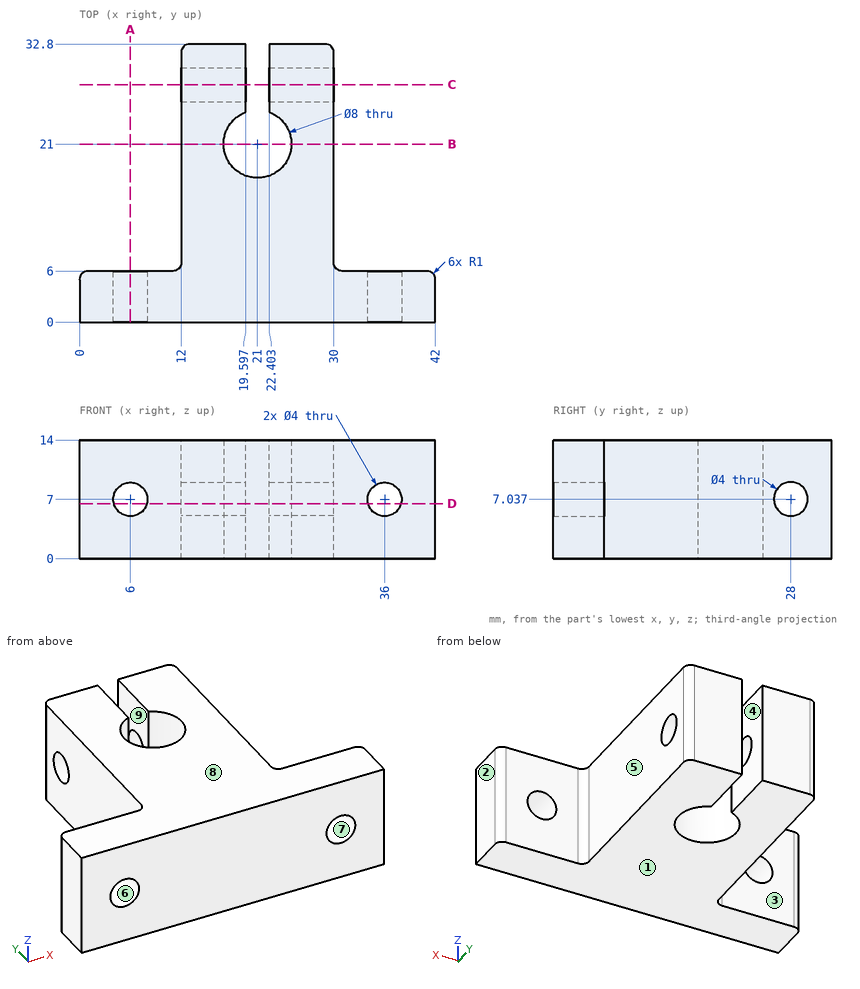
Print and shaded views of the part. All mm, measured from the part's lowest x, y and z. A direction names the side the tool comes from. Give positions to 0.01 mm unless a question says otherwise; leave off trailing zeros. Loops run counter-clockwise (first coordinate to the right, second up) from the corner with the lowest first, then second, coordinate; pieces in that order, holes last. Notation, with made-up numbers: M 4.25,-5 L 10.25,-5 A32 cw 10.25,28 Z; hole C 51,61 d1. An arc over 180 degrees is marked long. Write each question's results on one line, items separated by ' | '.
Q1. Band-saw the part on A-A on x = 6. Write the cut outline in (y, z), and give its area (3 significant figures).
Geometry check:
outline: M 0,0 L 6,0 L 6,5 L 0,5 Z; M 0,9 L 6,9 L 6,14 L 0,14 Z | area: 60.0 mm²
Q2. Mould opens along Z. For the marked faces 6, 7, 8 and 9 say: pulls with the +Z half, pulls with the -Z half, needs draft (parallel to the pull), parting line crosses it, or undercut.
Geometry check:
face 6: undercut | face 7: undercut | face 8: pulls with the +Z half | face 9: needs draft
Q3. Which spindle directions (+Z, -Z, +X, -X, +Y, -Y) get a long thin tool onto all of the face, cutting with end or side? Do the marked faces 1, 2, 3, 4 and 5. Say none if no direction does.
Geometry check:
face 1: -Z, +X, -X, +Y, -Y | face 2: +Z, -Z, +X, +Y, -Y | face 3: +Z, -Z, -X, +Y | face 4: +Z, -Z, +Y | face 5: +Z, -Z, +X, +Y
Q4. Flat gauge pins, fed straight in: P1, Ø8, axis at y = 18, z = 9, coming from the -X side; P2, Ø5, axis at x = 33.5, z = 8.5, coming from the +Y side; P3, Ø4.5, axis at y = 28, z = 7.04, coming from the +X side. Where does each tip first touch, or does it go through?
Geometry check:
P1: stops at x = 12 | P2: stops at y = 6 | P3: stops at x = 30
Q5. Band-saw the part on C-C on y = 28. Write the cut outline in (x, z), and give its area (3 significant figures).
Geometry check:
outline: M 12,0 L 19.6,0 L 19.6,5.04 L 12,5.04 Z; M 12,9.04 L 19.6,9.04 L 19.6,14 L 12,14 Z; M 22.4,0 L 30,0 L 30,5.04 L 22.4,5.04 Z; M 22.4,9.04 L 30,9.04 L 30,14 L 22.4,14 Z | area: 152 mm²
Q6. Band-saw the part on B-B on y = 21. Write the cut outline in (x, z).
Geometry check:
outline: M 12,0 L 17,0 L 17,14 L 12,14 Z; M 25,0 L 30,0 L 30,14 L 25,14 Z
Q7. Band-saw the part on D-D on z = 6.5. Give the number of separate pieces and of enclosed holes in the cut face.
Geometry check:
separate pieces: 5 | enclosed holes: 0
Q8. Probe probe 1 along X at (y, z) = (21, 10.5); probe 2 along Z at (x, y) = (6, 3.75); probe 3 along Y at (x, z) = (19, 7) (1 decimal). List the from-to ranges inside material, lowest first.
Geometry check:
probe 1: x = 12 to 17, 25 to 30 | probe 2: z = 0 to 5, 9 to 14 | probe 3: y = 0 to 17.5, 24.5 to 26, 30 to 32.8
